Design review of the part built by this model. Coordinates are the model's own, in mm. A direction names the side the tool comes from. Give positions to 0.01 mm unless a question says otherwise; leave off trailing zeros. Write each loop counter-clockwise with the first axis right and the second up, starting at its lowest first coordinate (ties: lowest second). Pieces come first, ordered by that corner, then holes. Notation, with made-up numbers: (-30, 13) -> (-22, 13) arc R18 cw to (-22, 43) -> close; hole circle Ø2 at (63, 45.25). An arc over 180 degrees is marked (long way). Use CSV: the item, a comma, the result in double quotes.
```python
from build123d import *

# Parameters (mm, degrees)
BOSS_EXTRUDE1_DEPTH = 17
CUT_EXTRUDE1_DEPTH  = 31
SKETCH3_W           = 12.47
SKETCH3_H           = 10.75
CUT_EXTRUDE2_REACH  = 25.639
SKETCH6_W           = 10
SKETCH6_H           = 10.75
SKETCH7_R           = 4
CUT_EXTRUDE3_DEPTH  = 31


with BuildPart() as part:
    # Sketch1 → Boss-Extrude1 (new body)
    with BuildSketch(Plane.XY):
        Polygon((0, 0), (0, 11.1), (5.04, 11.1), (5.04, -3.9), (-1.16650456, -19.86), (-6.626200647, -23.639063196), (-23.319289693, -8.973826134), (-26.37555014, -4.558379149), (-26.37555014, 11.1), (-21.33555014, 11.1), (-21.33555014, 0), align=None)
    extrude(amount=BOSS_EXTRUDE1_DEPTH)

    # Sketch2 → Cut-Extrude1 (cut, symmetric)
    with BuildSketch(Plane.ZY):
        Polygon((8.228054067, 11.1), (17, 11.1), (17, 12.88110255), (0, 12.88110255), (0, 11.1), align=None)
        with BuildLine():
            ThreePointArc((0, 0), (2.28131811, 6.908525055), (8.228054067, 11.1))
            Line((8.228054067, 11.1), (0, 11.1))
            Line((0, 11.1), (0, 0))
        make_face()
        Polygon((13.228054067, 10.512247596), (17, 6.76), (17, 11.1), (8.228054067, 11.1), align=None)
    extrude(amount=CUT_EXTRUDE1_DEPTH, both=True, mode=Mode.SUBTRACT)

    # Cut-Sweep1: sweep along a path in Sketch5
    with BuildLine(Plane.XY.offset(7)) as cut_sweep1_path:
        Line((-11.079626433, -19.726633046), (-3.773757644, -14.201247879))
    # Sketch3 → Cut-Sweep1 (sweep, cut)
    with BuildSketch(Plane(origin=(-14.60747623, -16.627341271, 0), x_dir=(-0.751264134, 0.660001668, 0), z_dir=(-0.660001668, -0.751264134, 0))):
        with Locations((-0.368794251, -9.115)):
            Rectangle(SKETCH3_W, SKETCH3_H)
    sweep(path=cut_sweep1_path.line, mode=Mode.SUBTRACT)

    # Cut-Extrude2: up to this face of the body (flat: up to its plane)
    cut_extrude2_end = Plane(part.part.faces().sort_by_distance((-5.99334807, -18.223163907, 9.115))[0])
    # Sketch6 → Cut-Extrude2 (cut, up to the picked face)
    with BuildSketch(Plane(origin=(0, 0, 0), x_dir=(1, 0, 0), z_dir=(0, 1, 0)), mode=Mode.PRIVATE) as cut_extrude2_sk1:
        with Locations((-8.42, -9.115)):
            Rectangle(SKETCH6_W, SKETCH6_H)
    cut_extrude2_tool1 = split(extrude(cut_extrude2_sk1.sketch, amount=-CUT_EXTRUDE2_REACH, mode=Mode.PRIVATE), bisect_by=cut_extrude2_end, keep=Keep.BOTH, mode=Mode.PRIVATE)
    add(cut_extrude2_tool1.solids().sort_by_distance((-8.42, 0, 9.115))[0], mode=Mode.SUBTRACT)

    # Sketch7 → Cut-Extrude3 (cut, symmetric)
    with BuildSketch(Plane.ZY.offset(10.66777507)):
        with Locations((8.5, 4.041620851)):
            Circle(SKETCH7_R)
    extrude(amount=CUT_EXTRUDE3_DEPTH, both=True, mode=Mode.SUBTRACT)


solid = part.part
```
(1) Clearance check with flat-ended pins moving along their axes: pin 1 (8.5 mm diameter, centred on x = -14.5, z = 11.5, fed in from +Y); pin 2 (2 mm diameter, centred on x = -1, z = 12.5, fed in from -Y); pin 3 (6.5 mm diameter, centred on y = 4.04, z = 8.5, fed in from +X); pin 4 (4 mm diameter, centred on y = -11.5, z = 7.5, fed in from -X). State where each tip first meets the part, or that it passes through.
Established:
pin 1,"stops at y = 0"
pin 2,"stops at y = -20.44"
pin 3,"passes through"
pin 4,"stops at x = -22.72"
(2) Take a section at D-D (x = -5). Write out the cut boundary in (y, z).
Established:
outline,"(-22.51, 0) -> (0, 0) -> (0, 3.74) -> (-17.47, 3.74) -> (-17.47, 14.49) -> (0, 14.49) -> (0, 17) -> (-22.51, 17) -> close"
(3) For line 1 along X through (y, z) = (-1.5, 9.25); line 2 along X through (y, z) = (1.5, 14.25); line 3 along Z through (x, y) = (-10, -10), list the stretches that pass through material, from the lowest coordinate up. Write a range as [from, to].
Established:
line 1,"x = [-26.38, -13.42], [-3.42, 5.04]"
line 2,"x = [-26.38, -21.34], [0, 5.04]"
line 3,"z = [0, 3.74], [14.49, 17]"
(4) Take a section at A-A (z = 6.25). Write out the cut boundary in (x, y), then the cut area to 3 significant figures.
Established:
outline,"(-26.38, -4.56) -> (-23.32, -8.97) -> (-19.01, -12.76) -> (-13.42, -8.52) -> (-13.42, 0) -> (-21.34, 0) -> (-21.34, 0.73) -> (-26.38, 0.73) -> close; (-26.38, 7.35) -> (-21.34, 7.35) -> (-21.34, 10.29) -> (-26.38, 10.29) -> close; (-9.65, -20.99) -> (-6.63, -23.64) -> (-1.17, -19.86) -> (5.04, -3.9) -> (5.04, 0.73) -> (0, 0.73) -> (0, 0) -> (-3.42, 0) -> (-3.42, -14.51) -> (-2.34, -15.46) -> close; (0, 7.35) -> (5.04, 7.35) -> (5.04, 10.29) -> (0, 10.29) -> close"
area,"307 mm2"
(5) Mouldability with a two-part tool opening along X and no side actions: class faces 1 (the face through (-24.826, -6.797, 8.381)), 2 (the face through (1.98, -11.77, 8.38)), 3 (the face through (-16, 0, 8)) as +X half, -X half, draft (parallel to the pull), parting line (faces both ways), or undercut.
Established:
face 1,"-X half"
face 2,"+X half"
face 3,"undercut"
(6) Take a section at B-B (y = -8). Write out the cut boundary in (x, z), then the cut area to 3 significant figures.
Established:
outline,"(-23.99, 0) -> (3.45, 0) -> (3.45, 17) -> (-23.99, 17) -> close; hole (-13.42, 3.74) -> (-3.42, 3.74) -> (-3.42, 14.49) -> (-13.42, 14.49) -> close"
area,"359 mm2"
(7) Tool access review of faces 4 (the face through (-2.873, -14.993, 9.04)), 5 (the face through (-16.18, -10.61, 9.19)), 6 (the face through (-13.42, -4, 9)), 7 (the face through (-9, -10, 3.74)): name each direction out of +Z, -Z, +X, -X, +Y, -Y from which nothing blocks a thin tool from reaching the whole face with its end or side.
Established:
face 4,"-X"
face 5,"-Y"
face 6,"+Y, -Y"
face 7,"none"
(8) Take a section at C-C (x = -22). Write out the cut boundary in (y, z).
Established:
outline,"(-10.13, 0) -> (0, 0) arc R11.6 ccw to (11.1, 8.23) -> (10.51, 13.23) -> (6.76, 17) -> (-10.13, 17) -> close; hole circle Ø8 at (4.04, 8.5)"
